Input: part model. Units: mm. Frame: model coordinates. A direction names the side the tool comes from. Coordinates: 2 decimals unless noted, no trailing zeros. Loops run counter-clockwise (first coordinate to the right, second up) from the corner with the lowest first, then second, coordinate; pieces in that order, holes last.
(1) Contact query for flat-ended pins moving along their axis: P1, Ø4, axis at y = -20.22, z = 18.25, coming from the +X side; P2, Ø0.8, axis at x = 64, z = 55, coming from the -Y side; P3, Ø0.8, axis at x = 63, y = -2, coming from the +Z side; P4, Ø0.5, axis at x = 64.5, y = -9, coming from the +Z side. Output: stop coordinate, or through.
(2) Section D-D, the plane x = -1.5. Return loops of the section in (y, z).
(3) Line query: L1, parallel to X at y = -20.75, z = 4; L2, parallel to Y at x = -28, z = 22. Output: solid intervals per line, ascending.
(4) Section C-C, the plane y = -24. Return loops of the section in (x, z).
(5) Section B-B, the plane z = 54.5. Return loops of the section in (x, y), then the cut area to 3 significant figures.
(6) Mould query, pull axis Z, two halves, no side actions, for faces 4 (the face through (64.064, -21.276, 16.865)), 5 (the face through (0.3, -0.5, 0)), 6 (the face through (-1, -1.016, 32)). Classes: released by +Z, released by -Z, zero draft, split by the parting line, or undercut.
(7) Set-up query: faces 1 (the face through (63.5, -1.1, 62.674)), 2 (the face through (-63.5, -1.1, 62.662)), 3 (the face through (63.564, -15, 24)). Return all of +Z, -Z, +X, -X, +Y, -Y with unobstructed straight access to the full face (end or side cutting, diameter ignored); none if empty.
(8) Section A-A, the plane y = -9.75. Return loops of the section in (x, z).
```python
from build123d import *

# Parameters (mm, degrees)
SKETCH1_W                       = 129.159
SKETCH1_H                       = 1.016
BASE_FLANGE1_DEPTH              = 64.262
EDGE_FLANGE1_STRIP_W            = 6.096
EDGE_FLANGE1_STRIP_H            = 1.016
EDGE_FLANGE1_STRIP_CUT_DEPTH    = 62.6745
EDGE_FLANGE1_RELIEF_W           = 6.8834
EDGE_FLANGE1_RELIEF_H           = 1.6002
EDGE_FLANGE1_RELIEF_CUT_DEPTH   = 1.016
EDGE_FLANGE1_STRIP_2_W          = 6.096
EDGE_FLANGE1_STRIP_2_H          = 1.016
EDGE_FLANGE1_STRIP_CUT_2_DEPTH  = 62.6618
EDGE_FLANGE1_RELIEF_2_W         = 6.8834
EDGE_FLANGE1_RELIEF_2_H         = 1.6002
EDGE_FLANGE1_RELIEF_CUT_2_DEPTH = 1.016
EDGE_FLANGE1_DEPTH              = 62.6745
EDGE_FLANGE1_BEND_DEPTH         = 62.6618
BREAK_CORNER1_START             = -64.5795
BREAK_CORNER1_DEPTH             = 129.159
F_1_8_0_125_DIAMETER_HOLE1_D    = 3.048
BREAK_CORNER2_START             = -1.016
BREAK_CORNER2_DEPTH             = 1.016
F_1_8_0_125_DIAMETER_HOLE4_D    = 3.4798
SKETCH20_W                      = 17.4625
SKETCH20_H                      = 24.1808
CUT_EXTRUDE4_DEPTH              = 148.065232295
CUT_EXTRUDE5_DEPTH              = 148.065232295
FILLET3_R                       = 1.5875


# Read off the part's stored shape, not the designer's step: Break-Corner1, Break-Corner2
# Sheet-metal steps are written as plain solids
with BuildPart() as part:
    # Sketch1 → Base-Flange1 (new body)
    with BuildSketch(Plane.XY):
        with Locations((0, -0.508)):
            Rectangle(SKETCH1_W, SKETCH1_H)
    extrude(amount=BASE_FLANGE1_DEPTH)

    # Edge-Flange1 strip (across the edge) → Edge-Flange1 strip cut (cut)
    with BuildSketch(Plane(origin=(64.5795, -1.016, 0), x_dir=(-1, 0, 0), z_dir=(0, 0, 1))):
        with Locations((-1.016, -0.508)):
            Rectangle(EDGE_FLANGE1_STRIP_W, EDGE_FLANGE1_STRIP_H)
    extrude(amount=EDGE_FLANGE1_STRIP_CUT_DEPTH, mode=Mode.SUBTRACT)

    # Edge-Flange1 relief (on the sheet) → Edge-Flange1 relief cut (cut)
    with BuildSketch(Plane(origin=(62.5475, -1.016, 0), x_dir=(-1, 0, 0), z_dir=(0, -1, 0))):
        with Locations((-2.6543, -63.4746)):
            Rectangle(EDGE_FLANGE1_RELIEF_W, EDGE_FLANGE1_RELIEF_H)
    extrude(amount=-EDGE_FLANGE1_RELIEF_CUT_DEPTH, mode=Mode.SUBTRACT)

    # Edge-Flange1 strip 2 (across the edge) → Edge-Flange1 strip cut 2 (cut)
    with BuildSketch(Plane(origin=(-64.5795, -1.016, 62.6618), x_dir=(1, 0, 0), z_dir=(0, 0, -1))):
        with Locations((-1.016, -0.508)):
            Rectangle(EDGE_FLANGE1_STRIP_2_W, EDGE_FLANGE1_STRIP_2_H)
    extrude(amount=EDGE_FLANGE1_STRIP_CUT_2_DEPTH, mode=Mode.SUBTRACT)

    # Edge-Flange1 relief 2 (on the sheet) → Edge-Flange1 relief cut 2 (cut)
    with BuildSketch(Plane(origin=(-62.5475, -1.016, 62.6618), x_dir=(1, 0, 0), z_dir=(0, -1, 0))):
        with Locations((-2.6543, 0.8001)):
            Rectangle(EDGE_FLANGE1_RELIEF_2_W, EDGE_FLANGE1_RELIEF_2_H)
    extrude(amount=-EDGE_FLANGE1_RELIEF_CUT_2_DEPTH, mode=Mode.SUBTRACT)

    # Edge-Flange1 section (across the edge) → Edge-Flange1 (add)
    with BuildSketch(Plane(origin=(64.5795, -1.016, 0), x_dir=(-1, 0, 0), z_dir=(0, 0, 1))):
        with BuildLine():
            Line((0, 1.016), (0, 27.559))
            Line((0, 27.559), (1.016, 27.559))
            Line((1.016, 27.559), (1.016, 1.016))
            ThreePointArc((1.016, 1.016), (1.31357951, 0.29757951), (2.032, 0))
            Line((2.032, 0), (2.032, -1.016))
            ThreePointArc((2.032, -1.016), (0.595159021, -0.420840979), (0, 1.016))
        make_face()
    extrude(amount=EDGE_FLANGE1_DEPTH)

    # Edge-Flange1 section 2 (across the edge) → Edge-Flange1 bend (add)
    with BuildSketch(Plane(origin=(-64.5795, -1.016, 62.6618), x_dir=(1, 0, 0), z_dir=(0, 0, -1))):
        with BuildLine():
            Line((0, 1.016), (0, 27.559))
            Line((0, 27.559), (1.016, 27.559))
            Line((1.016, 27.559), (1.016, 1.016))
            ThreePointArc((1.016, 1.016), (1.31357951, 0.29757951), (2.032, 0))
            Line((2.032, 0), (2.032, -1.016))
            ThreePointArc((2.032, -1.016), (0.595159021, -0.420840979), (0, 1.016))
        make_face()
    extrude(amount=EDGE_FLANGE1_BEND_DEPTH)

    # Break-Corner1 outline → Break-Corner1 (cut)
    with BuildSketch(Plane.YZ.offset(BREAK_CORNER1_START)):
        with BuildLine():
            ThreePointArc((-25.4, 0), (-27.64506403, 0.92993597), (-28.575, 3.175))
            Line((-28.575, 3.175), (-28.575, 0))
            Line((-28.575, 0), (-25.4, 0))
        make_face()
    extrude(amount=BREAK_CORNER1_DEPTH, mode=Mode.SUBTRACT)

    # 1/8 (0.125) Diameter Hole1 (through all)
    with Locations(Plane(origin=(64.5795, 0, 0), x_dir=(0, 0, -1), z_dir=(1, 0, 0))):
        with Locations((-4.7752, -6.746875)):
            Hole(F_1_8_0_125_DIAMETER_HOLE1_D / 2)

    # Break-Corner2 outline → Break-Corner2 (cut)
    with BuildSketch(Plane(origin=(0, 0, 0), x_dir=(1, 0, 0), z_dir=(0, 1, 0)).offset(BREAK_CORNER2_START)):
        with BuildLine():
            Line((-61.7601, -64.262), (-60.1726, -64.262))
            ThreePointArc((-60.1726, -64.262), (-61.295132015, -63.797032015), (-61.7601, -62.6745))
            Line((-61.7601, -62.6745), (-61.7601, -64.262))
        make_face()
        with BuildLine():
            ThreePointArc((61.7601, -62.6745), (61.295132015, -63.797032015), (60.1726, -64.262))
            Line((60.1726, -64.262), (61.7601, -64.262))
            Line((61.7601, -64.262), (61.7601, -62.6745))
        make_face()
    extrude(amount=BREAK_CORNER2_DEPTH, mode=Mode.SUBTRACT)

    # 1/8 (0.125) Diameter Hole4 (through all)
    with Locations(Plane(origin=(64.5795, 0, 0), x_dir=(0, 0, -1), z_dir=(1, 0, 0))):
        with Locations((-18.245584182, -20.217259182)):
            Hole(F_1_8_0_125_DIAMETER_HOLE4_D / 2)

    # Sketch20 → Cut-Extrude4 (cut, through all)
    with BuildSketch(Plane(origin=(64.5795, 0, 0), x_dir=(0, 0, -1), z_dir=(1, 0, 0))):
        with Locations((-53.94325, -16.4846)):
            Rectangle(SKETCH20_W, SKETCH20_H)
    extrude(amount=-CUT_EXTRUDE4_DEPTH, mode=Mode.SUBTRACT)

    # Sketch21 → Cut-Extrude5 (cut, through all)
    with BuildSketch(Plane(origin=(64.5795, 0, 0), x_dir=(0, 0, -1), z_dir=(1, 0, 0))):
        with BuildLine():
            Line((-39.806023342, -28.575), (-45.212, -28.575))
            Line((-45.212, -28.575), (-45.212, -15.022793726))
            ThreePointArc((-45.212, -15.022793726), (-43.112598411, -22.039667684), (-39.806023342, -28.575))
        make_face()
    extrude(amount=-CUT_EXTRUDE5_DEPTH, mode=Mode.SUBTRACT)

    # Fillet3
    fillet3_edges = [part.edges().sort_by_distance(p)[0] for p in [
        (64.0715, -4.3942, 62.6745),
        (-64.0715, -4.3942, 62.6618),
        (64.0715, -4.3942, 45.212),
        (-64.0715, -4.3942, 45.212),
        (64.0715, -15.022793726, 45.212),
        (64.0715, -28.575, 39.806023342),
        (-64.0715, -15.022793726, 45.212),
        (-64.0715, -28.575, 39.806023342),
    ]]
    fillet(fillet3_edges, radius=FILLET3_R)


solid = part.part
```
Report:
1. P1: stops at x = 64.58
1. P2: stops at y = -4.39
1. P3: passes through
1. P4: stops at z = 45.21
2. outline: (-1.02, 0) - (0, 0) - (0, 64.26) - (-1.02, 64.26) - close
3. L1: x = -64.58 to -63.56, 63.56 to 64.58
3. L2: y = -1.02 to 0
4. outline: (-64.58, 0) - (-63.56, 0) - (-63.56, 42.27) - (-64.58, 42.27) - close; (63.56, 0) - (64.58, 0) - (64.58, 42.27) - (63.56, 42.27) - close
5. outline: (-64.58, -4.39) - (-63.56, -4.39) - (-63.56, -2.03) arc R1.02 cw to (-62.55, -1.02) - (62.55, -1.02) arc R1.02 cw to (63.56, -2.03) - (63.56, -4.39) - (64.58, -4.39) - (64.58, -2.03) arc R2.03 ccw to (62.55, 0) - (-62.55, 0) arc R2.03 ccw to (-64.58, -2.03) - close
5. area: 137 mm2
6. face 4: undercut
6. face 5: released by -Z
6. face 6: zero draft
7. face 1: +Z, +X, +Y, -Y
7. face 2: +Z, -X, +Y, -Y
7. face 3: +Z, -Z, -Y
8. outline: (-64.58, 0) - (-63.56, 0) - (-63.56, 45.21) - (-64.58, 45.21) - close; (63.56, 0) - (64.58, 0) - (64.58, 45.21) - (63.56, 45.21) - close
